Autodesk Inventor part; units mm, degrees
ref_plane "YZ Plane" through (0, 0, 0) normal (1, 0, 0) x (0, 1, 0)
ref_plane "XZ Plane" through (0, 0, 0) normal (0, 1, 0) x (-1, 0, 0)
ref_plane "XY Plane" through (0, 0, 0) normal (0, 0, 1) x (1, 0, 0)
sketch "Sketch5" plane through (0, 0, 0) normal (0, 0, 1) x (1, 0, 0)
  circle A0 centre (0, 0) radius 5
  dimension "d8" = 10
extrude "Extrusion5" add sketch "Sketch5" along normal blind 19
hole "Hole2" at (0, 0, 19) direction (0, 0, -1) diameter 4.134 end through all
chamfer "Chamfer1" distance 1 angle 45 2 edges at (-5, 0, 19) (-5, 0, 0)
properties part number "BC-10026" material "Aço Carbono VC131"
CAD build for the part. Positions are in the model's coordinates, mm. Coordinates: 2 decimals unless noted, no trailing zeros. Order: outer loops, then holes, each group sorted by start corner. A loop starts at its lowest first (then second) coordinate and runs counter-clockwise, first axis right, second up. Notation, with made-up numbers: M 29.5,-36.75 L 44.5,-36.75 A13 cw 44.5,-25.75 Z; hole C -2.75,-39 d11. An arc over 180 degrees is marked long. Write each question's results on one line, items separated by ' | '. Start each with the question number.
Q1. Drill centre lines: probe 1 along Y at (x, z) = (0, 11); probe 2 along X at (y, z) = (-1, 3.75); probe 3 along Y at (x, z) = (0.5, 6.5). Where is each one in solid material? Low to high. Write a range as from..to.
Q2. Cut at C-C (z = 6.25). List the corners of the cut face in (x, y).
Q3. Cut at A-A (x = 0). List the corners of the cut face in (y, z), then the cut area to 3 significant figures.
Q4. Flat gauge pins, fed straight in: P1, Ø1.5, axis at x = -1, z = 3, coming from the -Y side; P2, Ø1, axis at x = 4, y = 2, coming from the +Z side; P3, Ø2, axis at y = 2, z = 9, coming from the -X side; P4, Ø1.5, axis at y = -2, z = 5, coming from the -X side. Where does each tip first touch, or does it go through?
Q5. Pull direction X, two halves, no side cores. Call faces 1 (the cylindrical face through (1.26, 1.64, 9.37)), 2 (the flat face through (2, -2, 0)), 3 (the cylindrical face through (-1.08, 4.88, 9.38)): +X half, -X half, draft (parallel to the pull), parting line (faces both ways), or undercut.
Found:
1) probe 1: -5..-2.07, 2.07..5 | probe 2: -4.9..-1.81, 1.81..4.9 | probe 3: -4.97..-2.01, 2.01..4.97
2) outline: C 0,0 d10; hole C 0,0 d4.13
3) outline: M -5,1 L -4,0 L -2.07,0 L -2.07,19 L -4,19 L -5,18 Z; M 2.07,0 L 4,0 L 5,1 L 5,18 L 4,19 L 2.07,19 Z | area: 109 mm²
4) P1: y = -4.99 | P2: z = 19 | P3: x = -4.9 | P4: x = -4.84
5) face 1: undercut | face 2: draft | face 3: parting line
